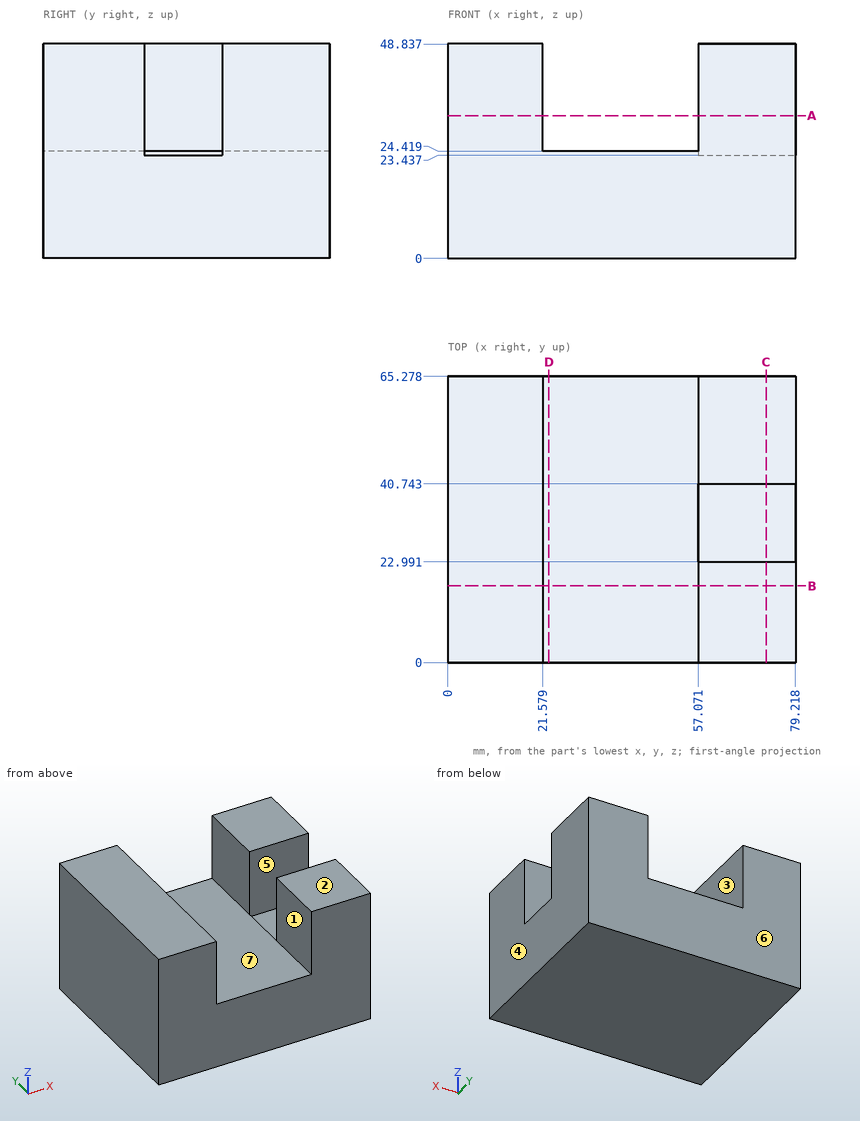
Input: dimensioned drawing with shaded views. Units: mm. Origin: part minimum x, y, z. A direction names the side the tool comes from. Give positions to 0.01 mm unless a question says otherwise; leave off trailing zeros. Order: outer loops, then holes, each group sorted by start corner. A loop starts at its lowest first (then second) coordinate and runs counter-clockwise, first axis right, second up. Notation, with made-up numbers: (32, 11.25) -> (82, 11.25) arc R6 cw to (82, 22.25) -> close; hole circle Ø3 at (-26, 12.5). An arc over 180 degrees is marked (long way). Write item = value, one per line.
Item 1: Set-up query: the marked faces 5, 6 and 7. Return all of +Z, -Z, +X, -X, +Y, -Y with unobstructed straight access to the full face (end or side cutting, diameter ignored); none if empty.
Check result:
face_5 = +Z, +X
face_6 = +Z, -Z, +X, -X, +Y
face_7 = +Z, +Y, -Y
Item 2: Mould query, pull axis X, two halves, no side actions, for the marked faces 1, 2, 3 and 4. Classes: +X half, -X half, draft (parallel to the pull), parting line (faces both ways), or undercut.
Check result:
face_1 = undercut
face_2 = draft
face_3 = undercut
face_4 = +X half
Item 3: Section query C-C (x = 72.5). Output: boundary loops of the cut face in (y, z).
Check result:
outline = (0, 0) -> (65.28, 0) -> (65.28, 48.84) -> (40.74, 48.84) -> (40.74, 23.44) -> (22.99, 23.44) -> (22.99, 48.84) -> (0, 48.84) -> close
Item 4: Section query D-D (x = 23). Output: boundary loops of the cut face in (y, z).
Check result:
outline = (0, 0) -> (65.28, 0) -> (65.28, 24.42) -> (0, 24.42) -> close
Item 5: Section query B-B (y = 17.5). Output: boundary loops of the cut face in (x, z).
Check result:
outline = (0, 0) -> (79.22, 0) -> (79.22, 48.84) -> (57.07, 48.84) -> (57.07, 24.42) -> (21.58, 24.42) -> (21.58, 48.84) -> (0, 48.84) -> close
Item 6: Contact query for flat-ended pins moving along their axis: pin 1 (5 mm diameter, centred on x = 25, y = 31.5, fed in from -Z); pin 2 (0.8 mm diameter, centred on y = 30, z = 24, fed in from +X); pin 3 (12 mm diameter, centred on x = 38.5, y = 45, fed in from +Z). Output: stop coordinate, or through.
Check result:
pin_1 = 0
pin_2 = 57.07
pin_3 = 24.42
Item 7: Section query A-A (z = 32.5). Output: boundary loops of the cut face in (x, y).
Check result:
outline = (0, 0) -> (21.58, 0) -> (21.58, 65.28) -> (0, 65.28) -> close; (57.07, 0) -> (79.22, 0) -> (79.22, 22.99) -> (57.07, 22.99) -> close; (57.07, 40.74) -> (79.22, 40.74) -> (79.22, 65.28) -> (57.07, 65.28) -> close
Item 8: Ray query, probe 1 along X at (y, z) = (3.5, 28); probe 2 along Z at (x, y) = (42, 48.5); probe 3 along X at (y, z) = (32.5, 28). Return the intervals inside material, ascending.
Check result:
probe_1 = 0 to 21.58, 57.07 to 79.22
probe_2 = 0 to 24.42
probe_3 = 0 to 21.58
